from build123d import *

# Parameters (mm, degrees)
F2_R        = 4.699
F3_DEPTH    = 9.525
F4_R        = 2.2225
F1_FACE_R   = 7.62
F1_FACE_R_2 = 4.699
F5_DEPTH    = 22.225


# Not quite as in the source:
# - a feature names something its author has since deleted; it is built from what else it names


with BuildPart() as f1:
    # F0 (on Front) → F1 (revolve)
    with BuildSketch(Plane.XZ):
        with BuildLine():
            ThreePointArc((11.0330758616, -81.8918719888), (13.2853990557, -80.4988733509), (15.6419463456, -79.2905315757))
            ThreePointArc((15.6419463456, -79.2905315757), (32.9902043329, -67.2816433685), (19.5133984089, -51.0473847389))
            ThreePointArc((19.5133984089, -51.0473847389), (13.498708034, -51.2466242985), (7.62, -52.533864975))
            Line((7.62, -52.533864975), (7.62, -44.9823363346))
            Line((7.62, -44.9823363346), (0, -44.9823363346))
            Line((0, -44.9823363346), (0, -88.1623363346))
            Line((0, -88.1623363346), (5.08, -88.1623363346))
            ThreePointArc((5.08, -88.1623363346), (5.7963291238, -86.1365407799), (7.512565547, -84.843672812))
            ThreePointArc((7.512565547, -84.843672812), (9.2048459257, -83.286701243), (11.0330758616, -81.8918719888))
        make_face()
    revolve(axis=Axis((0, 0, -66.5723363346), (0, 0, -1)))

    # F2 (on face) → F3 (cut)
    with BuildSketch(Plane.XY.offset(-44.9823363346)):
        Circle(F2_R)
    extrude(amount=-F3_DEPTH, mode=Mode.SUBTRACT)

    # F4 (on face) + F1_face (on face) → F5 (cut)
    with BuildSketch(Plane(origin=(0, 0, -88.1623363346), x_dir=(1, 0, 0), z_dir=(0, 0, -1))):
        Circle(F4_R)
    with BuildSketch(Plane.XY.offset(-44.9823363346)):
        Circle(F1_FACE_R)
        Circle(F1_FACE_R_2, mode=Mode.SUBTRACT)
    extrude(amount=-F5_DEPTH, dir=(0, 0, -1), mode=Mode.SUBTRACT)


solid = f1.part
The listing builds one solid part. Answer for the finished solid, in the listing's coordinates (mm). A direction names the side the tool comes from. Round coordinates to 2 decimals unless told otherwise and drop trailing zeros. Write each loop counter-clockwise with the first axis right and the second up, starting at its lowest first coordinate (ties: lowest second). Pieces come first, ordered by that corner, then holes. Notation, with made-up numbers: M 88.5,-9 L 146.5,-9 A17 ccw 146.5,8 Z; hole C 38.25,-9 d7. An arc over 180 degrees is marked long. Write each question's results on one line, items separated by ' | '. Start each with the question number.
Item 1: Given pin 1 Ø2 at (y, z) = (-16.5, -55) entering from -X; pin 2 Ø4 at (x, y) = (0, 0) entering from -Z; pin 3 Ø4.5 at (x, y) = (0, 1.5) entering from +Z, each flat-ended and moving along its own axis, determine where each tip first touches the part or whether it passes through.
Item 2: Find section C-C on z = -77.5. Write down the section's boundary in (x, y) (1 decimal), and give its area (3 significant figures).
Item 3: Find section A-A on z = -49. Write down the section's boundary in (x, y).
Item 4: Which of the six approach directions +Z, -Z, +X, -X, +Y, -Y give full straight-line access (tool end or side, diameter ignored) to faces 3 (the cylindrical face through (-0.61, 4.66, -49.68)), 4 (the flat face through (0, 0, -65.937)), 5 (the flat face through (-2.2, 1.1, -88.162))?
Item 5: Straight lines are drawn through the part: probe 1 along Z at (x, y) = (11, 16); probe 2 along Y at (x, z) = (-1, -53.5); probe 3 along X at (y, z) = (-2, -50). For each, find the intervals that lie inside material, in ascending order.
Item 6: Find section D-D on z = -55.5. Write down the section's boundary in (x, y).
Item 7: The mould has two halves that part along X. Classify faces 1 (the flat face through (0, 5, -44.982)), 2 (the flat face through (0, 0, -54.507)): +X half, -X half, draft (parallel to the pull), parting line (faces both ways), or undercut.
Item 8: Find section B-B on z = -64. Write down the section's boundary in (x, y).
Answer block:
1) pin 1: stops at x = -24.83 | pin 2: stops at z = -65.94 | pin 3: stops at z = -54.51
2) outline: C 0,0 d52.7; hole C 0,0 d4.4 | area: 2,170 mm²
3) outline: C 0,0 d15.24; hole C 0,0 d9.4
4) face 3: +Z | face 4: -Z | face 5: -Z, +X, -X, +Y, -Y
5) probe 1: z = -79.63 to -51.04 | probe 2: y = -26.83 to -4.59, 4.59 to 26.83 | probe 3: x = -7.35 to -4.25, 4.25 to 7.35
6) outline: C 0,0 d58.41
7) face 1: draft | face 2: undercut
8) outline: C 0,0 d66.12
